Here's how the part is built. I have some questions about the finished solid (model axes, mm). A direction names the side the tool comes from. Coordinates: 2 decimals unless noted, no trailing zeros. Write each loop counter-clockwise with the first axis right and the second up, starting at its lowest first coordinate (ties: lowest second). Pieces come first, ordered by that corner, then holes. Notation, with made-up numbers: M 80.5,80 L 109.5,80 A26 cw 109.5,117 Z; hole C 16.25,87.25 d10. An arc over 180 degrees is marked long. Use a Markdown table: item, result.
```python
from build123d import *

# Parameters (mm, degrees)
F0_W     = 133.35
F0_H     = 76.2
F2_DEPTH = 6.35
F1_W     = 50.8
F1_H     = 50.8
F1_W_2   = 45.466
F1_H_2   = 45.466
F3_DEPTH = 38.1
F4_START = -33.655
F4_DEPTH = 4.445


with BuildPart() as f2:
    # F0 (on Front) → F2 (new body)
    with BuildSketch(Plane.XZ):
        Rectangle(F0_W, F0_H)
    extrude(amount=-F2_DEPTH)

    # F1 (on Top) → F3 (join, symmetric)
    with BuildSketch(Plane.XY):
        with Locations((-28.575, -25.4)):
            Rectangle(F1_W, F1_H)
        with Locations((-28.575, -25.4)):
            Rectangle(F1_W_2, F1_H_2, mode=Mode.SUBTRACT)
        with Locations((28.575, -25.4)):
            Rectangle(F1_W, F1_H)
        with Locations((28.575, -25.4)):
            Rectangle(F1_W_2, F1_H_2, mode=Mode.SUBTRACT)
    extrude(amount=F3_DEPTH, both=True)

    # F1 (on Top) → F4 (join)
    with BuildSketch(Plane.XY.offset(F4_START)):
        with Locations((-28.575, -25.4)):
            Rectangle(F1_W_2, F1_H_2)
        with Locations((28.575, -25.4)):
            Rectangle(F1_W_2, F1_H_2)
    extrude(amount=-F4_DEPTH)


solid = f2.part
```
1. Suppose I cut it at B-B on y = -24. Write out the boundary of the cut face in (x, z) (3 decimals).
Answers follow:
| item | result |
|---|---|
| outline | M -53.975,-38.1 L -3.175,-38.1 L -3.175,38.1 L -5.842,38.1 L -5.842,-33.655 L -51.308,-33.655 L -51.308,38.1 L -53.975,38.1 Z; M 3.175,-38.1 L 53.975,-38.1 L 53.975,38.1 L 51.308,38.1 L 51.308,-33.655 L 5.842,-33.655 L 5.842,38.1 L 3.175,38.1 Z |
2. Suppose I cut it at A-A on z = 15. Write out the boundary of the cut face in (x, y) (3 decimals), and give its area (3 significant figures).
Answers follow:
| item | result |
|---|---|
| outline | M -66.675,0 L -53.975,0 L -53.975,-50.8 L -3.175,-50.8 L -3.175,0 L 3.175,0 L 3.175,-50.8 L 53.975,-50.8 L 53.975,0 L 66.675,0 L 66.675,6.35 L -66.675,6.35 Z; hole M -51.308,-48.133 L -5.842,-48.133 L -5.842,-2.667 L -51.308,-2.667 Z; hole M 5.842,-48.133 L 51.308,-48.133 L 51.308,-2.667 L 5.842,-2.667 Z |
| area | 1,870 mm2 |
3. Suppose I cut it at C-C on x = -41.5. Write out the boundary of the cut face in (y, z) (3 decimals), and give its area (3 significant figures).
Answers follow:
| item | result |
|---|---|
| outline | M -50.8,-38.1 L 6.35,-38.1 L 6.35,38.1 L -2.667,38.1 L -2.667,-33.655 L -48.133,-33.655 L -48.133,38.1 L -50.8,38.1 Z |
| area | 1,090 mm2 |
4. I need wall thicknesses on probe 1 along X at (y, z) = (-39, -21) (3 decimals); probe 2 along Y at (x, z) = (-30, -1); probe 3 along X at (y, z) = (-30, -35) (3 decimals). Which ranges of each line are inside material? Lowest first, please.
Answers follow:
| item | result |
|---|---|
| probe 1 | x = -53.975 to -51.308, -5.842 to -3.175, 3.175 to 5.842, 51.308 to 53.975 |
| probe 2 | y = -50.8 to -48.13, -2.67 to 6.35 |
| probe 3 | x = -53.975 to -3.175, 3.175 to 53.975 |
5. Which directions (+Z, -Z, +X, -X, +Y, -Y) give clear straight access to the entire face, cutting with the end or side of a thin tool? Please do faces 1 (the face through (28, -2.667, 3)), 2 (the face through (60, 0, 1)), 3 (the face through (-53.975, -26, -1)), 4 (the face through (3.175, -26, 1)).
Answers follow:
| item | result |
|---|---|
| face 1 | +Z |
| face 2 | +Z, -Z, +X, -Y |
| face 3 | +Z, -Z, -X, -Y |
| face 4 | +Z, -Z, -Y |
6. We'd pull the mould along X, two halves only. Please class faces 5 (the face through (53.975, -26, 1)), 6 (the face through (-51.308, -26, 2)), 7 (the face through (-60, 0, 1)), 8 (the face through (-29, -48.133, 2)): +X half, -X half, draft (parallel to the pull), parting line (faces both ways), or undercut.
Answers follow:
| item | result |
|---|---|
| face 5 | +X half |
| face 6 | undercut |
| face 7 | draft |
| face 8 | undercut |
7. Will these pins go through, and if not, where does the flat tip stop? pin 1 Ø13.5 at (y, z) = (-15, -15.5) entering from -X (3 decimals); pin 2 Ø5 at (x, y) = (18.5, -21) entering from +Z (3 decimals); pin 3 Ø1.9 at (x, z) = (-1, -3.5) entering from -Y.
Answers follow:
| item | result |
|---|---|
| pin 1 | stops at x = -53.975 |
| pin 2 | stops at z = -33.655 |
| pin 3 | stops at y = 0 |
